Check sheet for the modelled part. Datum: model origin and axes. Units: mm. A direction names the side the tool comes from. Coordinates: 2 decimals unless noted, no trailing zeros. Loops run counter-clockwise (first coordinate to the right, second up) from the corner with the lowest first, then second, coordinate; pieces in that order, holes last. Notation, with made-up numbers: (-16.5, 64) - (2.5, 64) arc R18 ccw to (2.5, 73) - close; hole circle Ø4 at (68.25, 5.5). An arc over 180 degrees is marked (long way). Write each question's results on one line, items separated by ' | '. Start each with the question number.
1. Tool access check on faces 1 (the face through (0, -5, 10)), 2 (the face through (-3, -7, 0)). Record the directions out of +Z, -Z, +X, -X, +Y, -Y that give a thin tool (end or side, any length) a straight path to the whole face; none if there is none.
2. Cross-section at C-C (z = -0.5). Record the cut outline in (x, y), and give its area (3 significant figures).
3. Thickness scan on line 1 (Y direction, x = 0, z = 7.5); line 2 (Z direction, x = -7.25, y = -1.5); line 3 (X direction, y = -0.5, z = 8.5). Record the ranges inside material, lowest first. Write a range as [from, to].
4. Gauge pin test, flat ends, axial feed: P1, Ø1, axis at x = -5.5, z = 0, coming from the -Y side; P2, Ø3, axis at x = -2.5, z = -2, coming from the -Y side; P3, Ø2, axis at x = 3, z = 3, coming from the -Y side. Record the tip position at first contact, or that the pin passes through.
5. Draft check along X on faces 3 (the face through (0, 0, -5)), 4 (the face through (0, 0, 0)), 5 (the face through (-8.87, 2.79, -2.46)). Enter one of: released by +X, released by -X, zero draft, split by the parting line, or undercut.
6. Cross-section at D-D (z = 3.5). Record the cut outline in (x, y), and give its area (3 significant figures).
7. Cross-section at A-A (x = 0). Record the cut outline in (y, z).
```python
from build123d import *

# Parameters (mm, degrees)
SKETCH1_R           = 7.217490794
SKETCH1_R_2         = 4.47
BOSS_EXTRUDE1_DEPTH = 10
SKETCH2_R           = 9.29699824
BOSS_EXTRUDE2_DEPTH = 5


with BuildPart() as part:
    # Sketch1 → Boss-Extrude1 (new body)
    with BuildSketch(Plane.XY):
        Circle(SKETCH1_R)
        Circle(SKETCH1_R_2, mode=Mode.SUBTRACT)
    extrude(amount=BOSS_EXTRUDE1_DEPTH)

    # Sketch2 → Boss-Extrude2 (add)
    with BuildSketch(Plane(origin=(0, 0, 0), x_dir=(-1, 0, 0), z_dir=(0, 0, -1))):
        Circle(SKETCH2_R)
    extrude(amount=BOSS_EXTRUDE2_DEPTH)


solid = part.part
```
Established:
1) face 1: +Z, +X, -X, +Y, -Y | face 2: +Z
2) outline: circle Ø18.59 at (0, 0) | area: 272 mm^2
3) line 1: [-7.22, -4.47], [4.47, 7.22] | line 2: [-5, 0] | line 3: [-7.2, -4.44], [4.44, 7.2]
4) P1: y = -7.84 | P2: y = -9.24 | P3: y = -6.93
5) face 3: zero draft | face 4: undercut | face 5: split by the parting line
6) outline: circle Ø14.43 at (0, 0); hole circle Ø8.94 at (0, 0) | area: 101 mm^2
7) outline: (-9.3, -5) - (9.3, -5) - (9.3, 0) - (7.22, 0) - (7.22, 10) - (4.47, 10) - (4.47, 0) - (-4.47, 0) - (-4.47, 10) - (-7.22, 10) - (-7.22, 0) - (-9.3, 0) - close
